Autodesk Fusion 360 part; units mm, degrees
sketch "Sketch1" plane through (0, 0, 0) normal (0, 0, 1) x (1, 0, 0)
  line L0 (0, 0) -> (19.5, 0)
  line L1 (19.5, 0) -> (19.5, 16)
  line L2 (19.5, 16) -> (0, 16)
  line L3 (0, 16) -> (0, 0)
  dimension "d1" = 19.5
  dimension "d2" = 16
extrude "Extrude1" add sketch "Sketch1" along normal blind 20
sketch "Sketch2" plane through (0, 0, 0) normal (0, -1, 0) x (1, 0, 0)
  line L0 (0, 0) -> (19.5, 0)
  line L1 (19.5, 0) -> (19.5, 20)
  line L2 (19.5, 20) -> (0, 20)
  line L3 (0, 20) -> (0, 0)
  line L4 (2, 0) -> (9, 0)
  line L5 (9, 0) -> (9, 5)
  line L6 (9, 5) -> (2, 5)
  line L7 (2, 5) -> (2, 0)
  dimension "d5" = 2
extrude "Extrude2" cut sketch "Sketch2" against normal blind 47 contours L0 L4 L5 L6 L7
sketch "Sketch3" plane through (0, 0, 20) normal (0, 0, 1) x (-1, 0, 0)
  line L0 (0, -16) -> (0, 0)
  line L1 (0, 0) -> (-19.5, 0)
  line L2 (-19.5, 0) -> (-19.5, -16)
  line L3 (-19.5, -16) -> (0, -16)
  line L4 (5, -8) -> (-24, -8) construction
  line L5 (-2, -13.5) -> (-15, -13.5)
  line L6 (-15, -13.5) -> (-15, -2.5)
  line L7 (-15, -2.5) -> (-2, -2.5)
  line L8 (-2, -2.5) -> (-2, -13.5)
  dimension "d8" = 8
  dimension "d9" = 13
  dimension "d10" = 11
  dimension "d11" = 2
  dimension "d12" = 5.5
extrude "Extrude3" cut sketch "Sketch3" against normal blind 36 contours L5 L6 L7 L8
sketch "Sketch4" plane through (19.5, 0, 0) normal (1, 0, 0) x (0, 1, 0)
  line L0 (0, 0) -> (16, 0)
  line L1 (16, 0) -> (16, 20)
  line L2 (16, 20) -> (0, 20)
  line L3 (0, 20) -> (0, 0)
  line L4 (5, 0) -> (9, 0)
  line L5 (9, 0) -> (9, 3)
  line L6 (9, 3) -> (5, 3)
  line L7 (5, 3) -> (5, 0)
extrude "Extrude4" cut sketch "Sketch4" against normal blind 8 contours L0 L4 L5 L6 L7
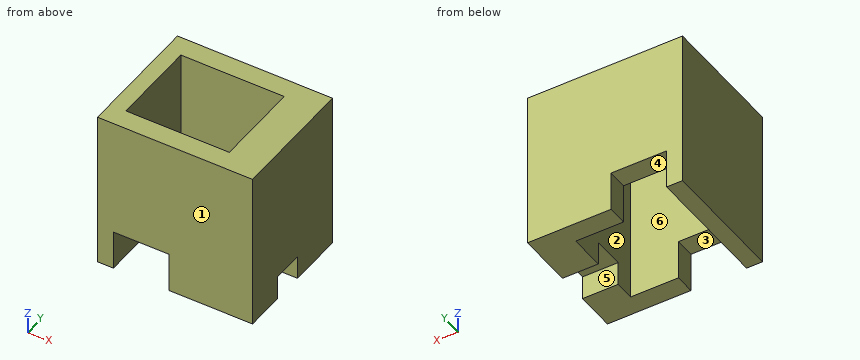
Here's how the part is built. I have some questions about the finished solid (model axes, mm). Face numbers are marked on the shaded views. A direction names the side the tool comes from. Give positions to 0.01 mm unless a question says otherwise; leave off trailing zeros. Loops run counter-clockwise (first coordinate to the right, second up) from the corner with the lowest first, then second, coordinate; pieces in that order, holes last. Notation, with made-up numbers: (48, 64) -> (59, 64) arc R8 cw to (59, 70) -> close; hole circle Ø3 at (4.25, 57). An arc over 180 degrees is marked (long way). Answer as a JSON object with one key per item and string values. Group by question number.
Item 1: Will this pin go through, and if not, where does the flat tip stop? pin 1 (1.2 mm diameter, centred on x = 6, y = 15.5, fed in from -Z).
Item 2: Imagine slicing it at D-D on y = 3. Write out the boundary of the cut face in (x, z).
Item 3: Imagine slicing it at C-C on z = 4.25. Write out the boundary of the cut face in (x, y), then the cut area to 3 significant figures.
Item 4: Imagine slicing it at A-A on x = 8. Write out the boundary of the cut face in (y, z).
Item 5: Thinking about a two-plate mould opening in Y: for the marked faces 1, 2 and 3, which applies, pulls with the +Y half, pulls with the -Y half, needs draft (parallel to the pull), parting line crosses it, or undercut?
Item 6: On a 3-axis mill with a long thin cutter (end or side, diameter ignored), from which of +Z, -Z, +X, -X, +Y, -Y can I reach the whole of each face in a straight line? I mean the marked faces 4, 5 and 6. Say none if no direction works.
Item 7: Imagine slicing it at B-B on z = 1.5. Write out the boundary of the cut face in (x, y).
Item 8: I need wall thicknesses on L1, parallel to Y at x = 7, z = 12.25; L2, parallel to X at y = 4, z = 1; L3, parallel to Z at x = 17, y = 7. Which ranges of each line are inside material? Lowest first, please.
Answer list:
{
 "1": {"pin 1": "stops at z = 5"},
 "2": {"outline": "(0, 0) -> (2, 0) -> (2, 20) -> (0, 20) -> close; (15, 0) -> (19.5, 0) -> (19.5, 20) -> (15, 20) -> close"},
 "3": {"outline": "(0, 0) -> (2, 0) -> (2, 16) -> (0, 16) -> close; (9, 0) -> (19.5, 0) -> (19.5, 16) -> (9, 16) -> (9, 13.5) -> (15, 13.5) -> (15, 2.5) -> (9, 2.5) -> close", "area": "134 mm2"},
 "4": {"outline": "(0, 5) -> (2.5, 5) -> (2.5, 20) -> (0, 20) -> close; (13.5, 5) -> (16, 5) -> (16, 20) -> (13.5, 20) -> close"},
 "5": {"face 1": "pulls with the -Y half", "face 2": "undercut", "face 3": "needs draft"},
 "6": {"face 4": "-Z, +Y, -Y", "face 5": "-Z, +X", "face 6": "+Z, -Z"},
 "7": {"outline": "(0, 0) -> (2, 0) -> (2, 16) -> (0, 16) -> close; (9, 0) -> (19.5, 0) -> (19.5, 5) -> (15, 5) -> (15, 2.5) -> (9, 2.5) -> close; (9, 13.5) -> (15, 13.5) -> (15, 9) -> (19.5, 9) -> (19.5, 16) -> (9, 16) -> close"},
 "8": {"L1": "y = 0 to 2.5, 13.5 to 16", "L2": "x = 0 to 2, 15 to 19.5", "L3": "z = 3 to 20"}
}
